from build123d import *

# Parameters (mm, degrees)
F0_R      = 11.1
F1_DEPTH  = 7
F2_SIZE   = 0.8
F3_R      = 12.5
F4_DEPTH  = 3
F5_R      = 12.5
F6_DEPTH  = 3
F8_R      = 22.5
F9_DEPTH  = 3
F10_R     = 22.5
F11_DEPTH = 3
F12_R     = 5
F13_DEPTH = 3
F14_R     = 5
F15_DEPTH = 3
F16_R     = 5
F17_DEPTH = 3
F18_R     = 5
F19_DEPTH = 3
F20_R     = 1.5
F21_R     = 2.5
F22_DEPTH = 25
F23_R     = 2.5
F24_DEPTH = 25
F25_SIZE  = 0.4
F26_SIZE  = 0.8
F27_W     = 103.2572649419
F27_H     = 49.3412911892
F28_DEPTH = 6.5


with BuildPart() as f1:
    # F0 (on Front) → F1 (new body)
    with BuildSketch(Plane.XZ):
        with BuildLine():
            ThreePointArc((21.7678643686, 14.8235294118), (-1.9380179843, 13), (-25.6439003372, 14.8235294118))
            ThreePointArc((-25.6439003372, 14.8235294118), (-42.9380179843, 0), (-25.6439003372, -14.8235294118))
            ThreePointArc((-25.6439003372, -14.8235294118), (-1.9380179843, -13), (21.7678643686, -14.8235294118))
            ThreePointArc((21.7678643686, -14.8235294118), (39.0619820157, 0), (21.7678643686, 14.8235294118))
        make_face()
        with Locations((-1.8380179843, 0)):
            Circle(F0_R, mode=Mode.SUBTRACT)
    extrude(amount=F1_DEPTH)

    # F2
    f2_edges = [f1.edges().sort_by_distance(p)[0] for p in [
        (-42.938018, -7, 0),
        (-1.938018, -7, -13),
        (-1.938018, 0, -13),
    ]]
    chamfer(f2_edges, length=F2_SIZE)

    # F3 (on face) → F4 (join)
    with BuildSketch(Plane.XZ.offset(7)):
        with Locations((-27.9380179843, 0)):
            Circle(F3_R)
        with Locations((24.0619820157, 0)):
            Circle(F3_R)
    extrude(amount=F4_DEPTH)

    # F5 (on face) → F6 (join)
    with BuildSketch(Plane(origin=(0, 0, 0), x_dir=(-1, 0, 0), z_dir=(0, 1, 0))):
        with Locations((-24.0619820157, 0)):
            Circle(F5_R)
        with Locations((27.9380179843, 0)):
            Circle(F5_R)
    extrude(amount=F6_DEPTH)

    # F8 (on face) → F9 (cut)
    with BuildSketch(Plane.XZ.offset(10)):
        with Locations((-1.8380179843, 0)):
            Circle(F8_R)
    extrude(amount=-F9_DEPTH, mode=Mode.SUBTRACT)

    # F10 (on face) → F11 (cut)
    with BuildSketch(Plane(origin=(0, 3, 0), x_dir=(-1, 0, 0), z_dir=(0, 1, 0))):
        with Locations((1.8380179843, 0)):
            Circle(F10_R)
    extrude(amount=-F11_DEPTH, mode=Mode.SUBTRACT)

    # F12 (on face) → F13 (cut)
    with BuildSketch(Plane(origin=(0, 3, 0), x_dir=(-1, 0, 0), z_dir=(0, 1, 0))):
        with Locations((-36.5619820157, 0)):
            Circle(F12_R)
    extrude(amount=-F13_DEPTH, mode=Mode.SUBTRACT)

    # F14 (on face) → F15 (cut)
    with BuildSketch(Plane(origin=(0, 3, 0), x_dir=(-1, 0, 0), z_dir=(0, 1, 0))):
        with Locations((40.4380179843, 0)):
            Circle(F14_R)
    extrude(amount=-F15_DEPTH, mode=Mode.SUBTRACT)

    # F16 (on face) → F17 (cut)
    with BuildSketch(Plane.XZ.offset(10)):
        with Locations((-40.4380179843, 0)):
            Circle(F16_R)
    extrude(amount=-F17_DEPTH, mode=Mode.SUBTRACT)

    # F18 (on face) → F19 (cut)
    with BuildSketch(Plane.XZ.offset(10)):
        with Locations((36.5617908537, 0)):
            Circle(F18_R)
    extrude(amount=-F19_DEPTH, mode=Mode.SUBTRACT)

    # F20
    f20_edges = [f1.edges().sort_by_distance(p)[0] for p in [
        (-39.438018, -8.5, 4.898979),
        (-39.438018, -8.5, -4.898979),
        (-21.592999, -8.5, -10.769899),
        (-21.592999, -8.5, 10.769899),
        (17.868739, -8.5, 10.857888),
        (17.868739, -8.5, -10.857888),
        (35.561967, -8.5, -4.899015),
        (35.561967, -8.5, 4.899015),
        (-21.592999, 1.5, -10.769899),
        (-21.592999, 1.5, 10.769899),
        (-39.438018, 1.5, 4.898979),
        (-39.438018, 1.5, -4.898979),
        (17.868739, 1.5, -10.857888),
        (17.868739, 1.5, 10.857888),
        (35.561982, 1.5, -4.898979),
        (35.561982, 1.5, 4.898979),
    ]]
    fillet(f20_edges, radius=F20_R)

    # F21 (on face) → F22 (cut)
    with BuildSketch(Plane.XZ.offset(7)):
        with Locations((-38.8380179843, 0)):
            Circle(F21_R)
    extrude(amount=-F22_DEPTH, mode=Mode.SUBTRACT)

    # F23 (on face) → F24 (cut)
    with BuildSketch(Plane.XZ.offset(7)):
        with Locations((34.9617908537, 0)):
            Circle(F23_R)
    extrude(amount=-F24_DEPTH, mode=Mode.SUBTRACT)

    # F25
    f25_edges = [f1.edges().sort_by_distance(p)[0] for p in [
        (-41.338018, -7, 0),
        (32.461791, -7, 0),
        (32.461791, 0, 0),
        (-41.338018, 0, 0),
    ]]
    chamfer(f25_edges, length=F25_SIZE)

    # F26
    f26_edges = [f1.edges().sort_by_distance(p)[0] for p in [
        (27.97166, -10, 11.872844),
        (18.498441, -10, 10.725925),
        (34.910055, -10, 5.322137),
        (20.661982, -10, 0),
        (31.561791, -10, 0),
        (18.498441, -10, -10.725925),
        (34.910055, -10, -5.322137),
        (27.97166, -10, -11.872844),
        (-24.338018, -10, 0),
        (-22.203581, -10, 10.646558),
        (-22.203581, -10, -10.646558),
        (-31.749718, -10, 11.904661),
        (-31.749718, -10, -11.904661),
        (-38.786142, -10, 5.322071),
        (-38.786142, -10, -5.322071),
        (-35.438018, -10, 0),
        (-24.338018, 3, 0),
        (-22.203581, 3, -10.646558),
        (-22.203581, 3, 10.646558),
        (-31.749718, 3, -11.904661),
        (-31.749718, 3, 11.904661),
        (-38.786142, 3, -5.322071),
        (-38.786142, 3, 5.322071),
        (-35.438018, 3, 0),
        (20.661982, 3, 0),
        (18.498441, 3, 10.725925),
        (18.498441, 3, -10.725925),
        (27.971709, 3, 11.872828),
        (27.971709, 3, -11.872828),
        (34.910106, 3, 5.322071),
        (34.910106, 3, -5.322071),
        (31.561982, 3, 0),
    ]]
    chamfer(f26_edges, length=F26_SIZE)

    # F27 (on face) → F28 (cut)
    with BuildSketch(Plane.XZ.offset(10)):
        with Locations((-3.2676365227, 0)):
            Rectangle(F27_W, F27_H)
    extrude(amount=-F28_DEPTH, mode=Mode.SUBTRACT)


solid = f1.part
Input: part model. Units: mm. Frame: model coordinates. A direction names the side the tool comes from. Round coordinates to 2 decimals unless told otherwise and drop trailing zeros. Use a Markdown table: item, result.
1. First-contact query: pin 1 (1 mm diameter, centred on x = -10.5, z = -7, fed in from +Y). Flat tip, straight axial feed; report the tip coordinate or a pass-through.
Evaluation:
| item | result |
|---|---|
| pin 1 | y = 0 |
2. Section A-A on z = 0. State how many separate pieces and enclosed holes the cut face has, then the cut area to 3 significant figures.
Evaluation:
| item | result |
|---|---|
| separate pieces | 4 |
| enclosed holes | 0 |
| area | 238 mm^2 |
3. Access query for faces 1 (the face through (27.854, 1.085, 11.911)), 2 (the face through (-24.338, 1.115, -0.137)), 3 (the face through (28.089, 1.085, -11.834)), 4 (the face through (-35.44, 1.12, 0.08)), 5 (the face through (-12, -3.5, -6)). Directions: +Z, -Z, +X, -X, +Y, -Y. A direction counts if a zero-diameter tool reaches every point of the face in a straight line with its end or side. Return the directions, or none.
Evaluation:
| item | result |
|---|---|
| face 1 | +Z, +Y |
| face 2 | +Y |
| face 3 | -Z, +Y |
| face 4 | -X, +Y |
| face 5 | +Z, -Z, +X, -X, -Y |
4. Material intervals for probe 1 along Y at (x, z) = (-19, -8.5); probe 2 along Z at (x, y) = (-11, -2.75); probe 3 along X at (y, z) = (-2, -10), sorted ascending.
Evaluation:
| item | result |
|---|---|
| probe 1 | -3.5 to 0 |
| probe 2 | -13.27 to -6.27, 6.27 to 13.27 |
| probe 3 | -39.12 to -6.66, 2.98 to 35.24 |
5. Mould query, pull axis Z, two halves, no side actions, for faces 6 (the face through (39.058, -2.131, -0.362)), 7 (the face through (20.8, 2.34, 0.14)), 8 (the face through (-2, -2, 13)). Classes: +Z half, -Z half, draft (parallel to the pull), parting line (faces both ways), or undercut.
Evaluation:
| item | result |
|---|---|
| face 6 | parting line |
| face 7 | undercut |
| face 8 | +Z half |
